Geometry: final body of the model. Coordinates: model frame, mm. Coordinates: 2 decimals unless noted, no trailing zeros. Order: outer loops, then holes, each group sorted by start corner. A loop starts at its lowest first (then second) coordinate and runs counter-clockwise, first axis right, second up. Notation, with made-up numbers: M 4,-17.5 L 26,-17.5 A14 cw 26,-0.5 Z; hole C -21,-21 d7. An arc over 180 degrees is marked long. Use CSV: the item, a comma, the result in double quotes. Start each with the question number.
1. Section query B-B on z = 5.5. Return the cut outline in (x, y), and give its area (3 significant figures).
2. Material intervals for line 1 (X direction, y = 1, z = 3); line 2 (Y direction, x = -7.5, z = -0.5); line 3 (Z direction, x = -14, y = 0.5), sorted ascending.
3. Section query D-D on x = -11. Return the cut outline in (y, z).
4. First-contact query: P1, Ø3, axis at y = 1, z = -2, coming from the +X side; P2, Ø1, axis at y = 1, z = 1, coming from the -X side; P3, Ø8, axis at x = 13, z = -8.5, coming from the -Y side; P4, Ø3, axis at x = -5.5, z = -7.5, coming from the +Y side. Flat tips, straight axial feed; report the tip coordinate or a pass-through.
5. Section query A-A on x = -2.5. Return the cut outline in (y, z), and give its area (3 significant figures).
6. Section query C-C on y = 5. Return the cut outline in (x, z) (3 decimals).
from build123d import *

# Parameters (mm, degrees)
BOSS_EXTRUDE2_DEPTH     = 1.27
SKETCH3_R               = 0.635
BOSS_EXTRUDE3_DEPTH     = 6.35
CUT_EXTRUDE1_DEPTH      = 6.35
CUT_EXTRUDE1_DEPTH_BACK = 6.35


with BuildPart() as part:
    # Sketch1 → Boss-Extrude2 (new body)
    with BuildSketch(Plane(origin=(0, 0, 0), x_dir=(1, 0, 0), z_dir=(0, 1, 0))):
        Polygon((7.62, -10.16), (-7.62, -10.16), (-7.62, 7.736503278), (-17.531075881, 7.736503278), (-17.531075881, 10.276503278), (-17.531075881, 12.816503278), (-16.261075881, 12.816503278), (-16.261075881, 10.16), (-16.261075881, 8.636), (-9.911075881, 8.636), (-9.911075881, 10.16), (-7.62, 10.16), (7.62, 10.16), (9.911075881, 10.16), (9.911075881, 8.636), (16.261075881, 8.636), (16.261075881, 10.16), (16.261075881, 12.816503278), (17.531075881, 12.816503278), (17.531075881, 10.276503278), (17.531075881, 7.736503278), (7.62, 7.736503278), align=None)
    extrude(amount=BOSS_EXTRUDE2_DEPTH)

    # Sketch3 → Boss-Extrude3 (add)
    with BuildSketch(Plane(origin=(0, 0, 0), x_dir=(1, 0, 0), z_dir=(0, 1, 0))):
        with Locations((-6.35, -8.89)):
            Circle(SKETCH3_R)
        with Locations((6.35, -8.89)):
            Circle(SKETCH3_R)
    extrude(amount=BOSS_EXTRUDE3_DEPTH)

    # Sketch4 → Cut-Extrude1 (cut, two sides)
    with BuildSketch(Plane(origin=(0, 0, 0), x_dir=(1, 0, 0), z_dir=(0, 1, 0))) as cut_extrude1_sk:
        with BuildLine():
            Line((3.81, -8.89), (-3.81, -8.89))
            ThreePointArc((-3.81, -8.89), (-5.606051224, -8.146051224), (-6.35, -6.35))
            Line((-6.35, -6.35), (-6.35, 6.35))
            ThreePointArc((-6.35, 6.35), (-5.606051224, 8.146051224), (-3.81, 8.89))
            Line((-3.81, 8.89), (3.81, 8.89))
            ThreePointArc((3.81, 8.89), (5.606051224, 8.146051224), (6.35, 6.35))
            Line((6.35, 6.35), (6.35, -6.35))
            ThreePointArc((6.35, -6.35), (5.606051224, -8.146051224), (3.81, -8.89))
        make_face()
    extrude(amount=CUT_EXTRUDE1_DEPTH, mode=Mode.SUBTRACT)
    extrude(cut_extrude1_sk.sketch, amount=-CUT_EXTRUDE1_DEPTH_BACK, mode=Mode.SUBTRACT)


solid = part.part
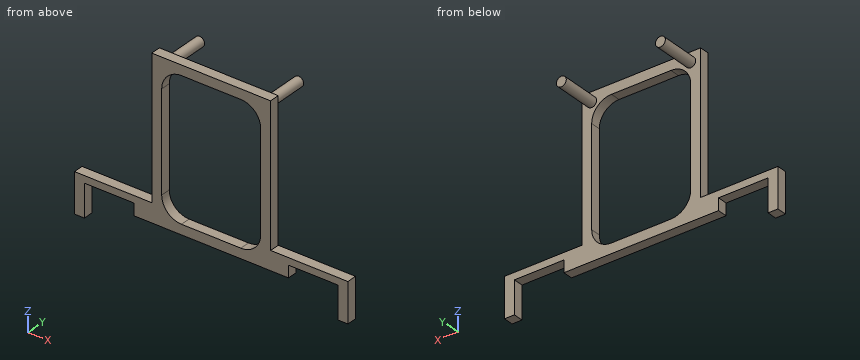
Results list:
1,outline,"M -7.62,0 L -6.35,0 L -6.35,1.27 L -7.62,1.27 Z; M 6.35,0 L 7.62,0 L 7.62,1.27 L 6.35,1.27 Z"
1,area,"3.23 mm²"
2,line 1,"x = -7.62 to -6.35, 6.35 to 7.62"
2,line 2,"y = 0 to 1.27"
2,line 3,"z = -8.64 to -7.74"
3,outline,"M 0,-8.64 L 1.27,-8.64 L 1.27,-7.74 L 0,-7.74 Z"
4,P1,"stops at x = 7.62"
4,P2,"stops at x = -7.62"
4,P3,"stops at y = 0"
4,P4,"stops at y = 1.27"
5,outline,"M 0,-10.16 L 1.27,-10.16 L 1.27,-8.89 L 0,-8.89 Z; M 0,8.89 L 1.27,8.89 L 1.27,10.16 L 0,10.16 Z"
5,area,"3.23 mm²"
6,outline,"C -6.35,8.89 d1.27; C 6.35,8.89 d1.27"
